Job drawing, mm, ordinate dimensions from the low corner. One solid piece. A direction names the side the tool comes from. Give positions to 0.01 mm unless a question says otherwise; leave off trailing zeros. Loops run counter-clockwise (first coordinate to the right, second up) from the corner with the lowest first, then second, coordinate; pieces in that order, holes last. Notation, with made-up numbers: (32.25, 29) -> (55.25, 29) arc R21 cw to (55.25, 62) -> close; hole circle Ø8 at (-20, 51.5). An arc over 180 degrees is marked (long way). Answer as a JSON object with one key per item and string values. Group by question number.
Q1. Two-plate mould, pull along Y, no slides. Class the marked faces 4, 5 and 6: pulls with the +Y half, pulls with the -Y half, needs draft (parallel to the pull), parting line crosses it, or undercut.
Q2. Band-saw the part on D-D, the plane y = 20. Write the cut outline in (x, z), plus the area to 3 significant figures.
Q3. Drop flat-ended pins along their axis: pin 1 (1.5 mm diameter, centred on x = 3, y = 36.5, fed in from -Z); pin 2 (20 mm diameter, centred on y = 25.4, z = 25.4, fed in from +X); pin 3 (8 mm diameter, centred on x = 4, y = 11.5, fed in from +Z). Give the stop position or say it passes through.
Q4. Band-saw the part on C-C, the plane x = 21.5. Write the cut outline in (y, z), plus the area to 3 significant figures.
Q5. Tool access for the marked faces 1, 2 and 3: list every direction of +Z, -Z, +X, -X, +Y, -Y with a clear straight run to the whole face (end or side of a thin tool).
Q6. Wall check: probe 1 along Z at (x, y) = (11.75, 25.4) (3 decimals); probe 2 along X at (y, z) = (23, 33); probe 3 along Y at (x, z) = (4.25, 26.5). Give the ranges that are in metal, low to high. Write a range as from..to.
Q7. Band-saw the part on A-A, the plane y = 25.4. Write the cut outline in (x, z) (1 decimal), plus the area to 3 significant figures.
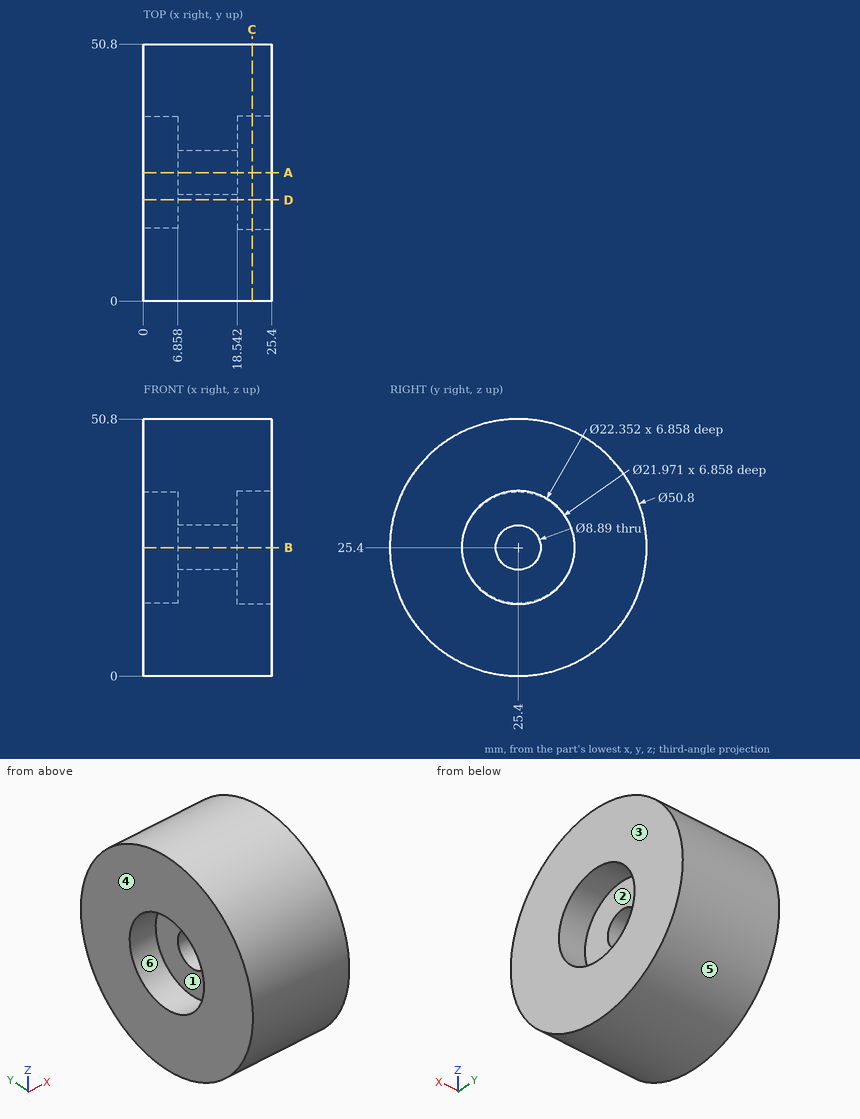
Worked answers:
{
 "1": {"face 4": "needs draft", "face 5": "parting line crosses it", "face 6": "undercut"},
 "2": {"outline": "(0, 0.58) -> (25.4, 0.58) -> (25.4, 15.62) -> (18.54, 15.62) -> (18.54, 35.18) -> (25.4, 35.18) -> (25.4, 50.22) -> (0, 50.22) -> (0, 34.97) -> (6.86, 34.97) -> (6.86, 15.83) -> (0, 15.83) -> close", "area": "995 mm2"},
 "3": {"pin 1": "z = 2.2", "pin 2": "x = 18.54", "pin 3": "z = 48.79"},
 "4": {"outline": "circle Ø50.8 at (25.4, 25.4); hole circle Ø22.35 at (25.4, 25.4)", "area": "1,630 mm2"},
 "5": {"face 1": "-X", "face 2": "+X", "face 3": "+Z, -Z, +X, +Y, -Y"},
 "6": {"probe 1": "0..20.955, 29.845..50.8", "probe 2": "6.86..18.54", "probe 3": "0.02..14.47, 36.33..50.78"},
 "7": {"outline": "(0, 0) -> (25.4, 0) -> (25.4, 14.2) -> (18.5, 14.2) -> (18.5, 21) -> (6.9, 21) -> (6.9, 14.4) -> (0, 14.4) -> close; (0, 36.4) -> (6.9, 36.4) -> (6.9, 29.8) -> (18.5, 29.8) -> (18.5, 36.6) -> (25.4, 36.6) -> (25.4, 50.8) -> (0, 50.8) -> close", "area": "882 mm2"}
}
